```python
from build123d import *

# Parameters (mm, degrees)
SKETCH2_R                             = 9.980949939
BOSS_EXTRUDE1_DEPTH                   = 44.45
F_1_4_20_TAPPED_HOLE1_D               = 5.1054
F_1_4_20_TAPPED_HOLE1_DEPTH           = 16.51
F_1_4_20_TAPPED_HOLE1_TIP             = 1.533816902
F_1_4_20_TAPPED_HOLE1_ON_FACE_2_D     = 5.1054
F_1_4_20_TAPPED_HOLE1_ON_FACE_2_DEPTH = 16.51
F_1_4_20_TAPPED_HOLE1_ON_FACE_2_TIP   = 1.533816902
F_1_4_20_TAPPED_HOLE1_ON_FACE_3_D     = 5.1054
F_1_4_20_TAPPED_HOLE1_ON_FACE_3_DEPTH = 16.51
F_1_4_20_TAPPED_HOLE1_ON_FACE_3_TIP   = 1.533816902
CHAMFER1_SIZE                         = 0.254


with BuildPart() as part:
    # Sketch2 → Boss-Extrude1 (new body, symmetric)
    with BuildSketch(Plane(origin=(0, 0, 0), x_dir=(0, 0, -1), z_dir=(1, 0, 0))):
        Circle(SKETCH2_R)
    extrude(amount=BOSS_EXTRUDE1_DEPTH, both=True)

    # 1/4-20 Tapped Hole1
    with Locations(Plane(origin=(-44.45, 0, 0), x_dir=(0, 0, -1), z_dir=(-1, 0, 0))):
        with Locations((0, 0)):
            Hole(F_1_4_20_TAPPED_HOLE1_D / 2, depth=F_1_4_20_TAPPED_HOLE1_DEPTH)
            with Locations((0, 0, -(F_1_4_20_TAPPED_HOLE1_DEPTH + F_1_4_20_TAPPED_HOLE1_TIP / 2))):  # 118° drill point
                Cone(0, F_1_4_20_TAPPED_HOLE1_D / 2, F_1_4_20_TAPPED_HOLE1_TIP, mode=Mode.SUBTRACT)

    # 1/4-20 Tapped Hole1 on face 2
    with Locations(Plane(origin=(14.956085126, -44.657762317, 0), x_dir=(0, 0, -1), z_dir=(-1, 0, 0))):
        with Locations((0, 0)):
            Hole(F_1_4_20_TAPPED_HOLE1_ON_FACE_2_D / 2, depth=F_1_4_20_TAPPED_HOLE1_ON_FACE_2_DEPTH)
            with Locations((0, 0, -(F_1_4_20_TAPPED_HOLE1_ON_FACE_2_DEPTH + F_1_4_20_TAPPED_HOLE1_ON_FACE_2_TIP / 2))):  # 118° drill point
                Cone(0, F_1_4_20_TAPPED_HOLE1_ON_FACE_2_D / 2, F_1_4_20_TAPPED_HOLE1_ON_FACE_2_TIP, mode=Mode.SUBTRACT)

    # 1/4-20 Tapped Hole1 on face 3
    with Locations(Plane(origin=(44.45, 0, 0), x_dir=(0, 0, 1), z_dir=(1, 0, 0))):
        with Locations((0, 0)):
            Hole(F_1_4_20_TAPPED_HOLE1_ON_FACE_3_D / 2, depth=F_1_4_20_TAPPED_HOLE1_ON_FACE_3_DEPTH)
            with Locations((0, 0, -(F_1_4_20_TAPPED_HOLE1_ON_FACE_3_DEPTH + F_1_4_20_TAPPED_HOLE1_ON_FACE_3_TIP / 2))):  # 118° drill point
                Cone(0, F_1_4_20_TAPPED_HOLE1_ON_FACE_3_D / 2, F_1_4_20_TAPPED_HOLE1_ON_FACE_3_TIP, mode=Mode.SUBTRACT)

    # Chamfer1
    chamfer1_edges = [part.edges().sort_by_distance(p)[0] for p in [
        (-44.45, 0, 9.980949939),
        (44.45, 0, 9.980949939),
        (-44.45, 0, -2.5527),
        (44.45, 0, 2.5527),
    ]]
    chamfer(chamfer1_edges, length=CHAMFER1_SIZE)


solid = part.part
```
Geometry: final body of the model. Coordinates: model frame, mm. A direction names the side the tool comes from. Round coordinates to 2 decimals unless told otherwise and drop trailing zeros. Order: outer loops, then holes, each group sorted by start corner. A loop starts at its lowest first (then second) coordinate and runs counter-clockwise, first axis right, second up. Notation, with made-up numbers: M 71,10 L 82,10 A35 cw 82,44 Z; hole C -34.5,-0.75 d6. An arc over 180 degrees is marked long. Use one line per item in the form item = value. Start each with the question number.
Q1. Cut plane B-B (x = 5.5). Return loops of the section in (y, z).
Q2. Mould query, pull axis Y, two halves, no side actions, for faces 4 (the face through (44.45, 2.3, -2)), 5 (the face through (0.619, -9.744, 2.164)), 6 (the face through (26.67, 0.39, 0.2)). Classes: +Y half, -Y half, draft (parallel to the pull), parting line (faces both ways), or undercut.
Q3. Pin query (flat end, axial travel): pin 1 Ø3 at (x, z) = (15, 3) entering from -Y; pin 2 Ø6 at (x, z) = (-23, 2) entering from +Y; pin 3 Ø8 at (x, y) = (-21, 4.5) entering from -Z; pin 4 Ø1.5 at (x, y) = (-11, -7) entering from +Z. Return the tip coordinate at first contact, or that it passes through.
Q4. Cut plane A-A (x = -34). Return loops of the section in (y, z), and give its area (3 significant figures).
Q5. Material intervals for line 1 (Y direction, x = -37.25, z = 0); line 2 (Z direction, x = 7.5, y = 0.5); line 3 (Y direction, x = -24, z = -2.25), sorted ascending. Write a range as [from, to].
Q6. Access query for faces 1 (the face through (35.954, -0.767, -2.435)), 2 (the face through (-35.954, -0.767, 2.435)), 3 (the face through (-44.45, 2.3, -2)). Directions: +Z, -Z, +X, -X, +Y, -Y. A direction counts if a zero-diameter tool reaches every point of the face in a straight line with its end or side. Return the directions, or none.
Geometry results:
q1.outline = C 0,0 d19.96
q2.face_4 = draft
q2.face_5 = parting line
q2.face_6 = undercut
q3.pin_1 = -9.87
q3.pin_2 = 9.98
q3.pin_3 = -9.97
q3.pin_4 = 7.78
q4.outline = C 0,0 d19.96; hole C 0,0 d5.11
q4.area = 292 mm^2
q5.line_1 = [-9.98, -2.55], [2.55, 9.98]
q5.line_2 = [-9.97, 9.97]
q5.line_3 = [-9.72, 9.72]
q6.face_1 = +X
q6.face_2 = -X
q6.face_3 = +Z, -Z, -X, +Y, -Y
